Can you work these out from the model? Positions are in its coordinate system, mm. Face numbers are marked on the shaded views. Coordinates: 2 decimals unless noted, no trailing zeros. Order: outer loops, then holes, each group sorted by start corner. A loop starts at its lowest first (then second) coordinate and runs counter-clockwise, first axis right, second up. Notation, with made-up numbers: (30.5, 16.5) -> (75.5, 16.5) arc R28 ccw to (75.5, 38.5) -> close; hole circle Ø4 at (69, 22). An arc over 180 degrees is marked (long way). Write item = value, one per line. Start each with the question number.
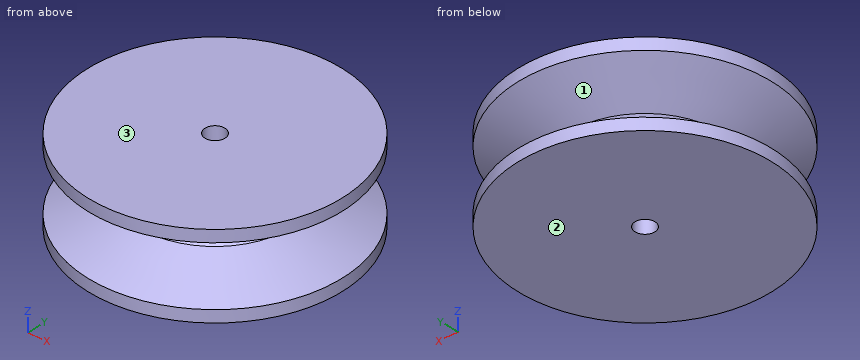
from build123d import *

# Parameters (mm, degrees)
F2_R     = 2.5
F3_DEPTH = 21


with BuildPart() as f1:
    # F0 (on Right) → F1 (revolve)
    with BuildSketch(Plane.YZ):
        Polygon((-160.7954752429, 0), (-128.7954752429, 0), (-128.7954752429, 21), (-160.7954752429, 21), (-160.7954752429, 18), (-147.9084072946, 12.5297642012), (-144.7954752429, 10.5), (-147.9084072946, 8.4702381086), (-160.7954752429, 3.0000023098), align=None)
    revolve(axis=Axis((0, -128.7954752429, 10.5), (0, 0, 1)))

    # F2 (on face) → F3 (cut, through all)
    with BuildSketch(Plane.XY.offset(21)):
        with Locations((0, -128.7954752429)):
            Circle(F2_R)
    extrude(amount=-F3_DEPTH, mode=Mode.SUBTRACT)


solid = f1.part
(1) For P1, Ø2, axis at x = 11, z = 17.5, coming from the -Y side; P2, Ø1, axis at y = -128.5, z = 19, coming from the -X side; P3, Ø8, axis at x = -21.5, z = 15, coming from the +Y side, each with a flat end and sliding along its axis, tell me the tip position at first contact or that it passes through.
(2) Imagine slicing it at C-C (z = 9.25). Write out the boundary of the cut face in (x, y).
(3) If I drill on L1, parallel to Z at x = 19.5, y = -150; L2, parallel to Z at x = -13, y = -145; L3, parallel to Y at x = 0, z = 13.25, over which ranges is the centre line in solid material (lowest first)? Write a range as from..to.
(4) Thinking about a two-plate mould opening in Z: for the marked faces 1, 2 and 3, which applies, +Z half, -Z half, draft (parallel to the pull), parting line (faces both ways), or undercut?
(5) Imagine slicing it at B-B (z = 4.75). Write out the boundary of the cut face in (x, y), plus the area to 3 significant figures.
(6) Imagine slicing it at A-A (x = 0). Write out the boundary of the cut face in (y, z), plus the area to 3 significant figures.
Result set:
q1.P1 = -159.15
q1.P2 = -32
q1.P3 = -102.94
q2.outline = circle Ø35.83 at (0, -128.8); hole circle Ø5 at (0, -128.8)
q3.L1 = 0..4.36, 16.64..21
q3.L2 = 0..7.76, 13.24..21
q3.L3 = -149.61..-131.3, -126.3..-107.99
q4.face_1 = undercut
q4.face_2 = -Z half
q4.face_3 = +Z half
q5.outline = circle Ø55.75 at (0, -128.8); hole circle Ø5 at (0, -128.8)
q5.area = 2,420 mm2
q6.outline = (-160.8, 0) -> (-131.3, 0) -> (-131.3, 21) -> (-160.8, 21) -> (-160.8, 18) -> (-147.91, 12.53) -> (-144.8, 10.5) -> (-147.91, 8.47) -> (-160.8, 3) -> close; (-126.3, 0) -> (-96.8, 0) -> (-96.8, 3) -> (-109.68, 8.47) -> (-112.8, 10.5) -> (-109.68, 12.53) -> (-96.8, 18) -> (-96.8, 21) -> (-126.3, 21) -> close
q6.area = 981 mm2
